Geometry check sheet. Reference: the model listing, model coordinates, mm. A direction names the side the tool comes from. Give positions to 0.01 mm unless a question says otherwise; leave off trailing zeros. Order: outer loops, then holes, each group sorted by start corner. A loop starts at its lowest first (then second) coordinate and runs counter-clockwise, first axis right, second up. Notation, with made-up numbers: M -38.5,-39.5 L -34.5,-39.5 A17 ccw -34.5,-33.5 Z; hole C 74.5,-36 d10. An arc over 180 degrees is marked long. Answer as CSV lines item,"result". Start each with the question number.
Q1. Section check C-C, the plane z = 1. Count the separate pieces of the cut face and the enclosed holes in it, then the cut area to 3 significant figures.
Q2. Set-up check for faces 1 (the cylindrical face through (19.73, 4.82, 1.31)), 2 (the flat face through (0, -101, -21.215)), 3 (the flat face through (-13, -59.565, 1)), 4 (the flat face through (0, -151.965, 16)), 5 (the cylindrical face through (0.28, -166.96, -1.54)): record each of +Z, -Z, +X, -X, +Y, -Y from which the full face is reachable in a straight line by a thin tool's end or side.
Q3. Section check A-A, the plane x = -4. Record the boundary of the cut face in (y, z) (3 decimals).
Q4. Section check B-B, the plane y = 33.5. Record the boundary of the cut face in (x, z) (3 decimals).
Q5. Go/stop test with flat-tipped pins: pin 1 (1.5 mm diameter, centred on x = -13.5, z = 2, fed in from -Y); pin 2 (1 mm diameter, centred on y = -99.5, z = 7.5, fed in from +X); pin 3 (1 mm diameter, centred on x = 24.5, z = -3.5, fed in from -Y); pin 4 (2.5 mm diameter, centred on x = 6, z = 0.5, fed in from -Y). Record where each tip stops, or that it passes through.
Q6. Section check D-D, the plane y = -83. Record the boundary of the cut face in (x, z) (3 decimals).
Q7. Thickness scan on line 1 (Z direction, x = 18, y = -49) (3 decimals); line 2 (X direction, y = -88, z = -2); line 3 (Y direction, x = 2.5, z = 14). Record the ranges inside material, lowest first.
```python
from build123d import *

# Parameters (mm, degrees)
SKETCH1_R           = 1.5
SKETCH1_R_2         = 8.5
BOSS_EXTRUDE1_DEPTH = 2.7
FILLET1_R           = 3
SCALE1_SCALE        = 1.9
BOSS_EXTRUDE2_START = -5.13
SKETCH2_W           = 22.8
SKETCH2_H           = 100
BOSS_EXTRUDE2_DEPTH = 20
SKETCH3_R           = 15
BOSS_EXTRUDE3_DEPTH = 22.8
CUT_EXTRUDE1_REACH  = 177.683
SKETCH4_R           = 5


with BuildPart() as part:
    # Sketch1 → Boss-Extrude1 (new body)
    with BuildSketch(Plane.XY):
        with BuildLine():
            Line((10.487675588, 31), (-10.487675588, 31))
            Line((-10.487675588, 31), (-20.108076211, 14.336977332))
            ThreePointArc((-20.108076211, 14.336977332), (-20.407777479, 13.613434467), (-20.51, 12.836977332))
            Line((-20.51, 12.836977332), (-20.51, -12.596152423))
            ThreePointArc((-20.51, -12.596152423), (-20.407777479, -13.372609558), (-20.108076211, -14.096152423))
            Line((-20.108076211, -14.096152423), (-10.348635262, -31))
            Line((-10.348635262, -31), (10.348635262, -31))
            Line((10.348635262, -31), (20.108076211, -14.096152423))
            ThreePointArc((20.108076211, -14.096152423), (20.407777479, -13.372609558), (20.51, -12.596152423))
            Line((20.51, -12.596152423), (20.51, 12.836977332))
            ThreePointArc((20.51, 12.836977332), (20.407777479, 13.613434467), (20.108076211, 14.336977332))
            Line((20.108076211, 14.336977332), (10.487675588, 31))
        make_face()
        with Locations(Location((-6, -27, 0), (0, 0, 180))):
            Circle(SKETCH1_R, mode=Mode.SUBTRACT)
        with Locations(Location((6, -27, 0), (0, 0, 180))):
            Circle(SKETCH1_R, mode=Mode.SUBTRACT)
        with Locations(Location((7.5, -13.4, 0), (0, 0, 180))):
            Circle(SKETCH1_R_2, mode=Mode.SUBTRACT)
        with BuildLine():
            ThreePointArc((-4.5, -13.4), (-8.54, -17.44), (-12.58, -13.4))
            Line((-12.58, -13.4), (-12.58, 1.685368783))
            ThreePointArc((-12.58, 1.685368783), (-10.18215631, 2.859423407), (-8.730303993, 5.1))
            Line((-8.730303993, 5.1), (8.729875369, 5.1))
            ThreePointArc((8.729875369, 5.1), (10.179804764, 2.860963681), (12.574584064, 1.685969643))
            ThreePointArc((12.574584064, 1.685969643), (14.121431526, -0.726790857), (11.622623122, -2.13039581))
            ThreePointArc((11.622623122, -2.13039581), (11.545720037, -2.104624526), (11.469942926, -2.075709596))
            ThreePointArc((11.469942926, -2.075709596), (0.558793877, -3.611248417), (-4.5, -13.4))
        make_face(mode=Mode.SUBTRACT)
        with Locations(Location((-13.5, 6.6, 0), (0, 0, 180))):
            Circle(SKETCH1_R, mode=Mode.SUBTRACT)
        with BuildLine():
            Line((8.729875369, 8.1), (-8.730303993, 8.1))
            ThreePointArc((-8.730303993, 8.1), (-10.179901517, 10.338575405), (-12.574074074, 11.513518208))
            ThreePointArc((-12.574074074, 11.513518208), (-0.00020804, 20.099999998), (12.57392263, 11.513905748))
            ThreePointArc((12.57392263, 11.513905748), (10.179553129, 10.338812856), (8.729875369, 8.1))
        make_face(mode=Mode.SUBTRACT)
        with Locations(Location((-5.24, 27, 0), (0, 0, 180))):
            Circle(SKETCH1_R, mode=Mode.SUBTRACT)
        with Locations(Location((13.5, 6.6, 0), (0, 0, 180))):
            Circle(SKETCH1_R, mode=Mode.SUBTRACT)
        with Locations(Location((5.24, 27, 0), (0, 0, 180))):
            Circle(SKETCH1_R, mode=Mode.SUBTRACT)
    extrude(amount=BOSS_EXTRUDE1_DEPTH)

    # Fillet1
    fillet1_edges = [part.edges().sort_by_distance(p)[0] for p in [
        (-10.487675588, 31, 1.35),
        (10.487675588, 31, 1.35),
        (10.348635262, -31, 1.35),
        (-10.348635262, -31, 1.35),
    ]]
    fillet(fillet1_edges, radius=FILLET1_R)


with BuildPart() as part_1:
    # Scale1: scaled about (-0.489793852, 0.73928426, 1.35)
    add(part.part.scale(SCALE1_SCALE).moved(Location((0.440814467, -0.665355834, -1.215))))

    # Sketch2 → Boss-Extrude2 (add, symmetric)
    with BuildSketch(Plane.XY.offset(3.915).offset(BOSS_EXTRUDE2_START)):
        with Locations((0.440814467, -101.965355834)):
            Rectangle(SKETCH2_W, SKETCH2_H)
    extrude(amount=BOSS_EXTRUDE2_DEPTH, both=True)

    # Sketch3 → Boss-Extrude3 (add)
    with BuildSketch(Plane.ZY.offset(10.959185533)):
        with Locations((-1.215, -151.965355834)):
            Circle(SKETCH3_R)
    extrude(amount=-BOSS_EXTRUDE3_DEPTH)

    # Sketch4 → Cut-Extrude1 (cut, up to next)
    with BuildSketch(Plane(origin=(11.840814467, 0, 0), x_dir=(0, 0, -1), z_dir=(1, 0, 0)), mode=Mode.PRIVATE) as cut_extrude1_sk1:
        with Locations(Location((1.215, -151.965355834, 0), (0, 0, 90))):
            Circle(SKETCH4_R)
    cut_extrude1_tool1 = extrude(cut_extrude1_sk1.sketch, amount=-CUT_EXTRUDE1_REACH, mode=Mode.PRIVATE) & part_1.part
    add(cut_extrude1_tool1.solids().sort_by_distance((11.840814, -151.965356, -1.215))[0], mode=Mode.SUBTRACT)


solid = part_1.part
```
Answer block:
1,separate pieces,"2"
1,enclosed holes,"9"
1,area,"7,270 mm2"
2,face 1,"+Z, -Z"
2,face 2,"-Z, +X, -X, +Y, -Y"
2,face 3,"+Z, -Z, -X, -Y"
2,face 4,"+Z, +X, -X, -Y"
2,face 5,"+X, -X, -Y"
3,outline,"M -151.965,-21.215 L -51.965,-21.215 L -51.965,-1.215 L -13.068,-1.215 L -13.068,3.915 L -51.965,3.915 L -51.965,18.785 L -151.965,18.785 L -151.965,13.785 A15 ccw -151.965,-16.215 Z; M 9.025,-1.215 L 14.725,-1.215 L 14.725,3.915 L 9.025,3.915 Z; M 37.137,-1.215 L 58.235,-1.215 L 58.235,3.915 L 37.137,3.915 Z; hole C -151.965,-1.215 d10"
4,outline,"M -33.766,-1.215 L -13.353,-1.215 L -13.353,3.915 L -33.766,3.915 Z; M 14.235,-1.215 L 34.648,-1.215 L 34.648,3.915 L 14.235,3.915 Z"
5,pin 1,"stops at y = -59.57"
5,pin 2,"stops at x = 11.84"
5,pin 3,"passes through"
5,pin 4,"stops at y = -166.96"
6,outline,"M -10.959,-21.215 L 11.841,-21.215 L 11.841,18.785 L -10.959,18.785 Z"
7,line 1,"z = -1.215 to 3.915"
7,line 2,"x = -10.96 to 11.84"
7,line 3,"y = -151.97 to -51.97"
